Job drawing, mm, ordinate dimensions from the low corner. One solid piece. A direction names the side the tool comes from. Round coordinates to 2 decimals unless told otherwise and drop trailing zeros. Loops run counter-clockwise (first coordinate to the right, second up) from the corner with the lowest first, then second, coordinate; pieces in that order, holes last. Notation, with made-up numbers: M -30,39.5 L -6,39.5 A13 ccw -6,49.5 Z; hole C 4,-15 d2. An arc over 180 degrees is marked long. Use one line per item in the form item = value.
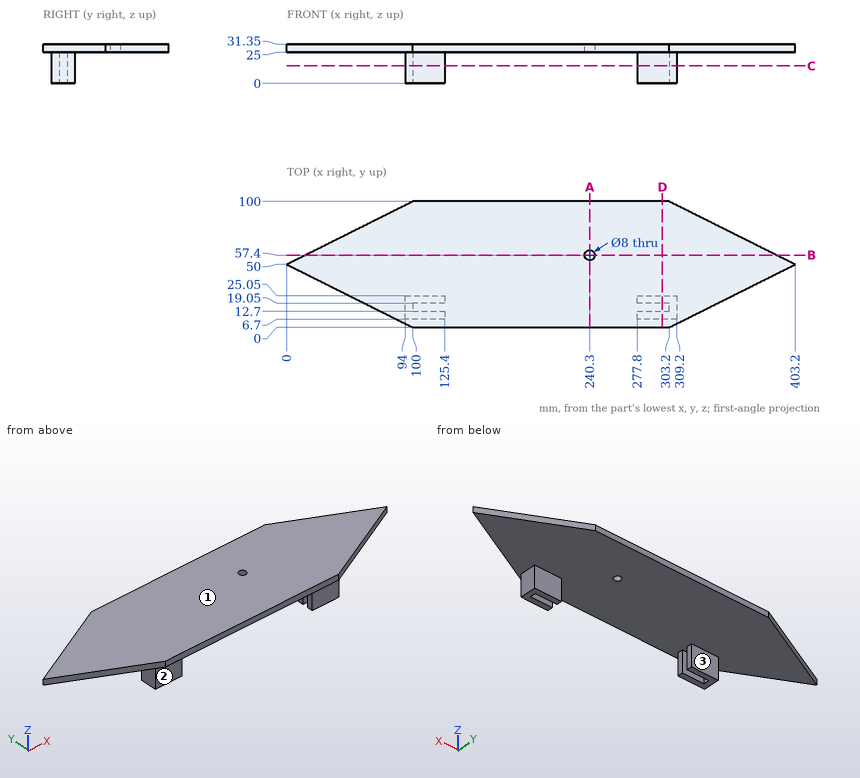
1. Cut at D-D on x = 298. Write the cut outline in (y, z).
Completed:
outline = M 0,25 L 6.7,25 L 6.7,0 L 12.7,0 L 12.7,25 L 19.05,25 L 19.05,0 L 25.05,0 L 25.05,25 L 100,25 L 100,31.35 L 0,31.35 Z
2. Probe line 1 along Y through (x, z) = (240.3, 27.25); line 2 along Z through (x, y) = (116, 38.5); line 3 along X through (y, z) = (57, 26). List the from-to ranges inside material, lowest first. Write a range as from..to.
Completed:
line_1 = 0..53.4, 61.4..100
line_2 = 25..31.35
line_3 = 14..236.32, 244.28..389.2
3. Cut at A-A on x = 240.3. Write the cut outline in (y, z).
Completed:
outline = M 0,25 L 53.4,25 L 53.4,31.35 L 0,31.35 Z; M 61.4,25 L 100,25 L 100,31.35 L 61.4,31.35 Z
4. Drop flat-ended pins along their axis: P1, Ø1, axis at x = 93, y = 82.5, coming from the -Z side; P2, Ø2, axis at y = 20, z = 14.5, coming from the +X side; P3, Ø9, axis at y = 17.5, z = 6.5, coming from the -X side. Give the stop position or say it passes through.
Completed:
P1 = 25
P2 = 309.2
P3 = 94
5. Cut at C-C on z = 14. Write the cut outline in (x, y), and give its area (3 significant figures).
Completed:
outline = M 94,6.7 L 125.4,6.7 L 125.4,12.7 L 100,12.7 L 100,19.05 L 125.4,19.05 L 125.4,25.05 L 94,25.05 Z; M 277.8,6.7 L 309.2,6.7 L 309.2,25.05 L 277.8,25.05 L 277.8,19.05 L 303.2,19.05 L 303.2,12.7 L 277.8,12.7 Z
area = 830 mm2
6. Cut at B-B on y = 57.4. Write the cut outline in (x, z).
Completed:
outline = M 14.8,25 L 236.3,25 L 236.3,31.35 L 14.8,31.35 Z; M 244.3,25 L 388.4,25 L 388.4,31.35 L 244.3,31.35 Z
7. Tool access for the marked faces 1, 2 and 3: list every direction of +Z, -Z, +X, -X, +Y, -Y with a clear straight run to the whole face (end or side of a thin tool).
Completed:
face_1 = +Z, +X, -X, +Y, -Y
face_2 = -Z, +X, -X, -Y
face_3 = -Z, +X, -X, +Y
